from build123d import *

# Parameters (mm, degrees)
F0_W      = 44.1574328202
F0_H      = 45.3486293554
F1_DEPTH  = 25.4
F2_DEPTH  = 12.7
F3_W      = 44.1574328202
F3_H      = 16.4641523734
F4_DEPTH  = 50.8
F5_W      = 15.0199290365
F5_H      = 19.4511728585
F6_DEPTH  = 50.8
F8_DEPTH  = 10.16
F10_DEPTH = 50.8


with BuildPart() as f1:
    # F0 (on Top) → F1 (new body)
    with BuildSketch(Plane.XY):
        Rectangle(F0_W, F0_H)
        with BuildLine():
            Line((22.0787164101, -22.6743146777), (-22.0787164101, -22.6743146777))
            ThreePointArc((-22.0787164101, -22.6743146777), (0, -44.7530310878), (22.0787164101, -22.6743146777))
        make_face()
    extrude(amount=F1_DEPTH)

    # F2 (cut): a face of the model
    f2_faces = [f1.faces().sort_by_distance(p)[0] for p in [
        (0, -8.8639771544, 25.4),
    ]]
    extrude(f2_faces, amount=-F2_DEPTH, mode=Mode.SUBTRACT)

    # F3 (on face) → F4 (join)
    with BuildSketch(Plane.XY.offset(12.7)):
        with Locations((0, 14.442238491)):
            Rectangle(F3_W, F3_H)
    extrude(amount=F4_DEPTH)

    # F5 (on face) → F6 (cut)
    with BuildSketch(Plane.XZ.offset(-6.2101623043)):
        with Locations((-0.1444215886, 53.7744135708)):
            Rectangle(F5_W, F5_H)
        with BuildLine():
            Line((7.3655429296, 44.0488271415), (-7.6543861069, 44.0488271415))
            ThreePointArc((-7.6543861069, 44.0488271415), (-0.1444215886, 35.7909022145), (7.3655429296, 44.0488271415))
        make_face()
    extrude(amount=-F6_DEPTH, mode=Mode.SUBTRACT)

    # F7 (on face) → F8 (cut)
    with BuildSketch(Plane.YZ.offset(22.0787164101)):
        Polygon((-8.2320761867, 0), (22.6743146777, 0), (22.6743146777, 22.0966245979), (6.2101623043, 22.0966245979), (6.2101623043, 12.7), (-8.2320761867, 12.7), align=None)
    extrude(amount=-F8_DEPTH, mode=Mode.SUBTRACT)

    # F9 (on face) → F10 (cut)
    with BuildSketch(Plane.XY.offset(12.7)):
        with BuildLine():
            Line((22.0787164101, -8.2320761867), (16.9987164101, -8.2320761867))
            Line((16.9987164101, -8.2320761867), (16.9987164101, -28.7400558591))
            Line((16.9987164101, -28.7400558591), (21.229142758, -28.7400558591))
            ThreePointArc((21.229142758, -28.7400558591), (21.8652914559, -25.7367888192), (22.0787164101, -22.6743146777))
            Line((22.0787164101, -22.6743146777), (22.0787164101, -8.2320761867))
        make_face()
    extrude(amount=-F10_DEPTH, mode=Mode.SUBTRACT)


solid = f1.part
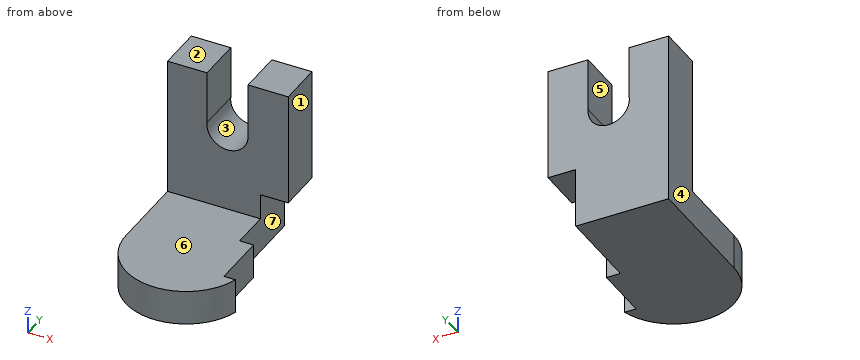
Input: part model. Units: mm. Frame: model coordinates. Face numbers are marked on the shaded views. A direction names the side the tool comes from. Coordinates: 2 decimals unless noted, no trailing zeros. Order: outer loops, then holes, each group sorted by start corner. A loop starts at its lowest first (then second) coordinate and runs counter-clockwise, first axis right, second up. Notation, with made-up numbers: M -15,32.25 L 0,32.25 A19 ccw 0,42.25 Z; hole C 11.25,-22.75 d10. An arc over 180 degrees is marked long. Write item = value, one per line. Start each with the question number.
(1) Section C-C on y = 11.5. Output: boundary loops of the cut face in (x, z), and give its area (3 significant figures).
(2) Section D-D on x = 13. Output: boundary loops of the cut face in (y, z), and give its area (3 significant figures).
(3) Line query: line 1 along X through (y, z) = (7, 54); line 2 along Y through (x, z) = (-6, 33); line 3 along Z through (x, y) = (-1, -40). Output: solid intervals per line, ascending. Write a range as [from, to].
(4) Section A-A on z = 52. Output: boundary loops of the cut face in (x, y), and give its area (3 significant figures).
(5) Pull-direction query (X, two-part tool) for the marked faces 1, 2, 3 and 4; classes: released by +X, released by -X, zero draft, split by the parting line, or undercut.
(6) First-contact query: P1, Ø5, axis at y = -12.5, z = 13, coming from the +X side; P2, Ø8, axis at x = 19, y = 10.5, coming from the -Z side; P3, Ø19.5, axis at x = -0.14, z = 43.33, coming from the -Y side; P4, Ø12, axis at y = -11, z = 20.5, coming from the +X side. Flat tips, straight axial feed; report the tip coordinate or a pass-through.
(7) Reachability of the marked faces 5, 6 and 7 from +Z, -Z, +X, -X, +Y, -Y: full face, straight path, thin tool, end or side. Return the list, or none.
(8) Section B-B on z = 8. Output: boundary loops of the cut face in (x, y).
Result set:
q1.outline = M -22.08,0 L 11.92,0 L 11.92,22.1 L 22.08,22.1 L 22.08,63.5 L 7.37,63.5 L 7.37,44.05 A7.54 cw long -7.65,44.05 L -7.65,63.5 L -22.08,63.5 Z
q1.area = 2,190 mm²
q2.outline = M -40.52,0 L -8.23,0 L -8.23,12.7 L -40.52,12.7 Z; M 6.21,22.1 L 22.67,22.1 L 22.67,63.5 L 6.21,63.5 Z
q2.area = 1,090 mm²
q3.line_1 = [-22.08, -7.65], [7.37, 22.08]
q3.line_2 = [6.21, 22.67]
q3.line_3 = [0, 12.7]
q4.outline = M -22.08,6.21 L -7.65,6.21 L -7.65,22.67 L -22.08,22.67 Z; M 7.37,6.21 L 22.08,6.21 L 22.08,22.67 L 7.37,22.67 Z
q4.area = 480 mm²
q5.face_1 = released by +X
q5.face_2 = zero draft
q5.face_3 = undercut
q5.face_4 = released by -X
q6.P1 = 17
q6.P2 = 22.1
q6.P3 = 6.21
q6.P4 = through
q7.face_5 = +Z, +Y, -Y
q7.face_6 = +Z, +X, -X, -Y
q7.face_7 = -Z, +X, +Y
q8.outline = M -22.08,-22.67 A22.08 ccw 21.23,-28.74 L 17,-28.74 L 17,-8.23 L 11.92,-8.23 L 11.92,22.67 L -22.08,22.67 Z
